```python
from build123d import *

# Parameters (mm, degrees)
RECTANGLE003_W     = 9
RECTANGLE003_H     = 9
EXTRUSION005_DEPTH = 2
CIRCLE_R           = 4.26
EXTRUSION001_DEPTH = 34.920666
RECTANGLE_W        = 28.2
RECTANGLE_H        = 58
EXTRUSION_DEPTH    = 2


with BuildPart() as extrusion005:
    # Rectangle003 (on Cut) → Extrusion005 (new body)
    with BuildSketch(Plane(origin=(-284.476256, -56.100832, -3.133948), x_dir=(1, 0, 0), z_dir=(0, 0, 1))):
        with Locations((4.5, 4.5)):
            Rectangle(RECTANGLE003_W, RECTANGLE003_H)
    extrude(amount=-EXTRUSION005_DEPTH)


with BuildPart() as extrusion001:
    # Circle → Extrusion001 (new body)
    with BuildSketch(Plane(origin=(-279.976256, -51.600832, -5.133948), x_dir=(0, 1, 0), z_dir=(0, 0, -1))):
        Circle(CIRCLE_R)
    extrude(amount=-EXTRUSION001_DEPTH)


with BuildPart() as cut002:
    # Rectangle → Extrusion (new body)
    with BuildSketch(Plane(origin=(-309.476256, -65.700832, -5.133948), x_dir=(0, 1, 0), z_dir=(0, 0, -1))):
        with Locations((14.1, 29)):
            Rectangle(RECTANGLE_W, RECTANGLE_H)
    extrude(amount=-EXTRUSION_DEPTH)

    # Cut: cut Extrusion001
    add(extrusion001.part, mode=Mode.SUBTRACT)

    # Cut002: cut Extrusion005
    add(extrusion005.part, mode=Mode.SUBTRACT)


solid = cut002.part
```
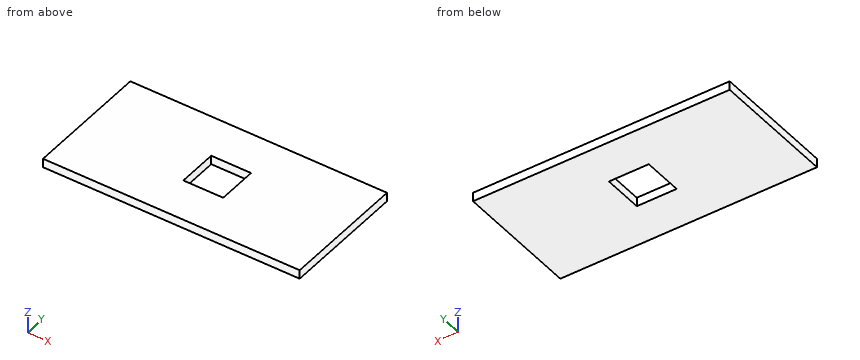
CAD build for the part. Positions are in the model's coordinates, mm. Give positions to 0.01 mm unless a question says otherwise; leave off trailing zeros. Order: outer loops, then holes, each group sorted by start corner. A loop starts at its lowest first (then second) coordinate and runs counter-clockwise, first axis right, second up.
(1) Saw through at B-B, the plane z = -3.6. Give the cut face in (x, y).
(2) Drill centre lines: L1, parallel to X at y = -49.5, z = -4.1; L2, parallel to Y at x = -282.5, z = -4.45. Where is each one in solid material? Low to high.
(3) Saw through at A-A, the plane y = -48. Give the cut face in (x, z), then the cut area to 3 significant figures.
Results found:
1. outline: (-309.48, -65.7) - (-251.48, -65.7) - (-251.48, -37.5) - (-309.48, -37.5) - close; hole (-284.48, -56.1) - (-275.48, -56.1) - (-275.48, -47.1) - (-284.48, -47.1) - close
2. L1: x = -309.48 to -284.48, -275.48 to -251.48
2. L2: y = -65.7 to -56.1, -47.1 to -37.5
3. outline: (-309.48, -5.13) - (-284.48, -5.13) - (-284.48, -3.13) - (-309.48, -3.13) - close; (-275.48, -5.13) - (-251.48, -5.13) - (-251.48, -3.13) - (-275.48, -3.13) - close
3. area: 98.0 mm2
